Input: dimensioned drawing with shaded views. Units: mm. Origin: part minimum x, y, z. Coordinates: 2 decimals unless noted, no trailing zeros. Write each loop counter-clockwise with the first axis right and the second up, starting at its lowest first coordinate (ties: lowest second). Pieces come first, ordered by that corner, then holes. Notation, with made-up numbers: (44, 8.5) - (50, 8.5) arc R27 ccw to (50, 31.5) - close; hole circle Ø3 at (84, 85.25). An arc over 180 degrees is marked (long way). One line per question, with ' | ' between items.
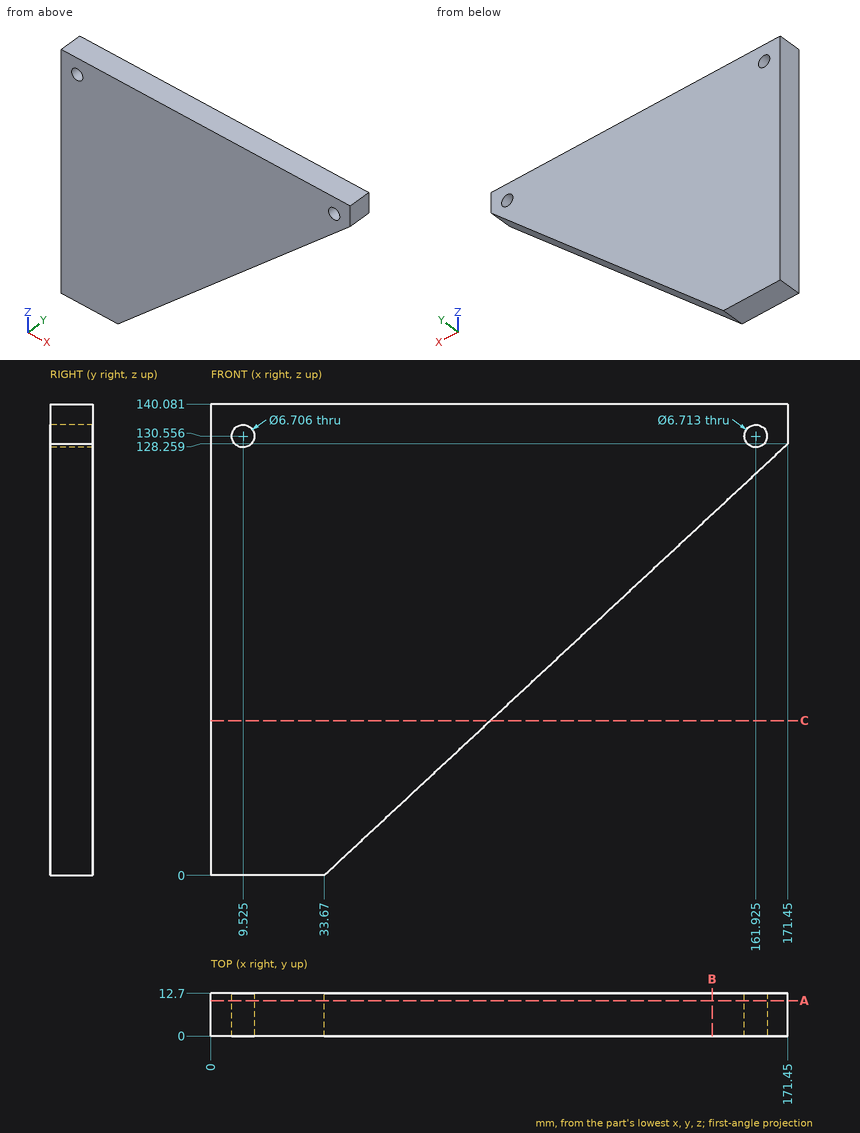
Item 1: Cut plane C-C on z = 46. Return loops of the section in (x, y) (1 decimal), and give its area (3 significant figures).
Check sheet entries:
outline: (0, 0) - (83.1, 0) - (83.1, 12.7) - (0, 12.7) - close | area: 1,060 mm²
Item 2: Cut plane A-A on y = 10.5. State how many separate pieces and enclosed holes the cut face has, and give its area (3 significant figures).
Check sheet entries:
separate pieces: 1 | enclosed holes: 2 | area: 15,100 mm²
Item 3: Ray query, line 1 along Z through (x, y) = (9, 5) (1 decimal); line 2 along X through (y, z) = (1.25, 26.5) (1 decimal); line 3 along Z through (x, y) = (156, 2.5) (1 decimal). Return the intervals inside material, ascending. Write a range as [from, to].
Check sheet entries:
line 1: [0, 127.2], [133.9, 140.1] | line 2: [0, 62.1] | line 3: [113.9, 140.1]
Item 4: Cut plane B-B on x = 149. Return loops of the section in (y, z).
Check sheet entries:
outline: (0, 107.36) - (12.7, 107.36) - (12.7, 140.08) - (0, 140.08) - close
Item 5: Pin query (flat end, axial travel): pin 1 Ø3 at (y, z) = (5.5, 38) entering from +X; pin 2 Ø3 at (x, y) = (116, 3.5) entering from -Z (1 decimal); pin 3 Ø1 at (y, z) = (3.5, 41) entering from +X. Return the tip coordinate at first contact, or that it passes through.
Check sheet entries:
pin 1: x = 76.1 | pin 2: z = 75.2 | pin 3: x = 78.25
